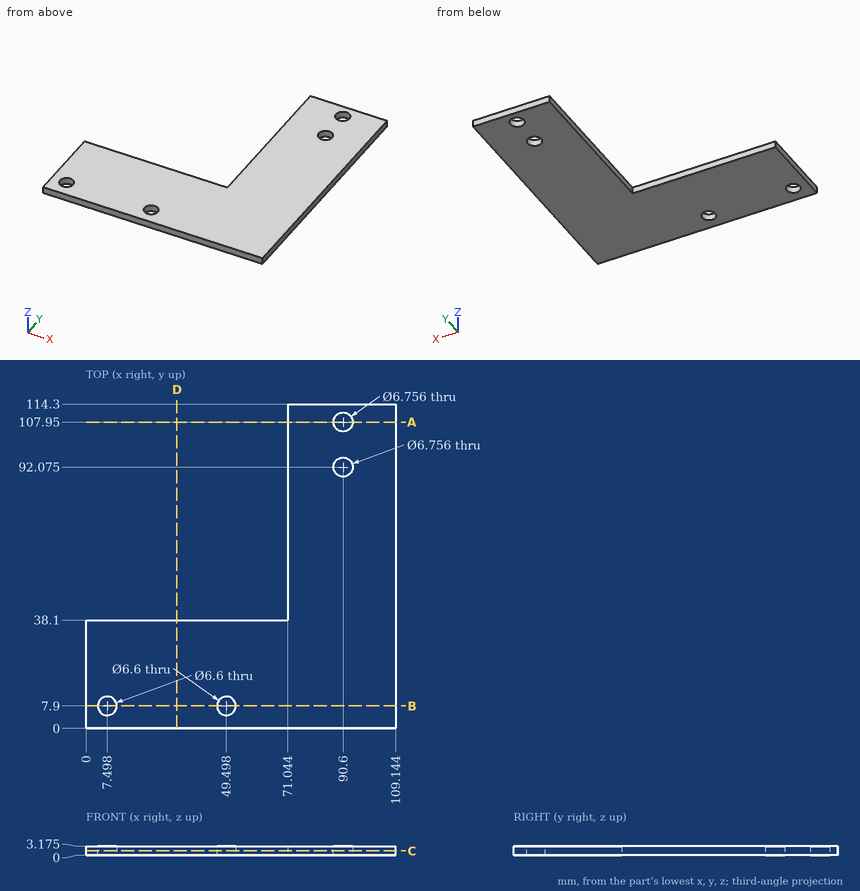
Answer from the drawing. Dimensions are ordinates in mm from the lowest x, y and z of the part. Coordinates: 2 decimals unless noted, no trailing zeros. Loops run counter-clockwise (first coordinate to the right, second up) from the corner with the lowest first, then second, coordinate; pieces in that order, holes last. Notation, with made-up numbers: (57.5, -26) -> (71.5, -26) arc R7 cw to (71.5, -15) -> close; hole circle Ø6 at (12.25, 85.5). An arc over 180 degrees is marked (long way). Answer as CSV lines item,"result".
Q1. The part is cut by section A-A on y = 107.95. Write down the section's boundary in (x, z) (1 decimal).
Findings:
outline,"(71, 0) -> (87.2, 0) -> (87.2, 3.2) -> (71, 3.2) -> close; (94, 0) -> (109.1, 0) -> (109.1, 3.2) -> (94, 3.2) -> close"
Q2. The part is cut by section D-D on x = 32. Write down the section's boundary in (y, z) (1 decimal), and give its area (3 significant figures).
Findings:
outline,"(0, 0) -> (38.1, 0) -> (38.1, 3.2) -> (0, 3.2) -> close"
area,"121 mm²"
Q3. The part is cut by section B-B on y = 7.9. Write down the section's boundary in (x, z) (1 decimal).
Findings:
outline,"(0, 0) -> (4.2, 0) -> (4.2, 3.2) -> (0, 3.2) -> close; (10.8, 0) -> (46.2, 0) -> (46.2, 3.2) -> (10.8, 3.2) -> close; (52.8, 0) -> (109.1, 0) -> (109.1, 3.2) -> (52.8, 3.2) -> close"
Q4. The part is cut by section C-C on z = 1.6. State how many separate pieces and enclosed holes the cut face has, and give its area (3 significant figures).
Findings:
separate pieces,"1"
enclosed holes,"4"
area,"6,920 mm²"
Q5. This flat-tipped pin is pushed along its axis until it touches: pin 1 (1 mm diameter, centred on y = 77.5, z = 0.5, fed in from -X). Where does it stop, or does it pass through?
Findings:
pin 1,"stops at x = 71.04"
Q6. Find the intervals of material crossed by probe 1 along Y at (x, z) = (88.5, 0.5) (1 decimal); probe 2 along X at (y, z) = (69, 3); probe 3 along Y at (x, z) = (57, 2.45), in increasing order.
Findings:
probe 1,"y = 0 to 89.4, 94.7 to 105.3, 110.6 to 114.3"
probe 2,"x = 71.04 to 109.14"
probe 3,"y = 0 to 38.1"
